from build123d import *

# Parameters (mm, degrees)
SKETCH_1_R      = 1.65
EXTRUDE_1_DEPTH = 1.6
EXTRUDE_2_DEPTH = 4.8
EXTRUDE_3_DEPTH = 0.01


with BuildPart() as part:
    # 草图1 → 凸台-拉伸1 (new body)
    with BuildSketch(Plane(origin=(0, 0, 0), x_dir=(1, 0, 0), z_dir=(0, 1, 0))):
        with BuildLine():
            Line((27.181335969, 0), (83.591335969, 0))
            Line((83.591335969, 0), (83.591335969, 96.2))
            Line((83.591335969, 96.2), (78.265479271, 96.2))
            ThreePointArc((78.265479271, 96.2), (76.9576214, 96.598857266), (76.026335969, 97.6))
            Line((76.026335969, 97.6), (55.386335969, 97.6))
            Line((55.386335969, 97.6), (34.746335969, 97.6))
            ThreePointArc((34.746335969, 97.6), (33.815050539, 96.598857266), (32.507192668, 96.2))
            Line((32.507192668, 96.2), (27.181335969, 96.2))
            Line((27.181335969, 96.2), (27.181335969, 0))
        make_face()
        with Locations(Location((31.021335969, 2.73, 0), (0, 0, 270))):
            Circle(SKETCH_1_R, mode=Mode.SUBTRACT)
        with Locations(Location((79.751335969, 2.73, 0), (0, 0, 90))):
            Circle(SKETCH_1_R, mode=Mode.SUBTRACT)
    extrude(amount=EXTRUDE_1_DEPTH)

    # 草图3 → 凸台-拉伸2 (add)
    with BuildSketch(Plane(origin=(0, 1.6, 0), x_dir=(1, 0, 0), z_dir=(0, 1, 0))):
        Polygon((55.386335969, 7), (27.886335969, 7), (27.886335969, 91.7), (82.886335969, 91.7), (82.886335969, 7), align=None)
    extrude(amount=EXTRUDE_2_DEPTH)

    # 草图4 → 凸台-拉伸3 (add)
    with BuildSketch(Plane(origin=(0, 6.4, 0), x_dir=(1, 0, 0), z_dir=(0, 1, 0))):
        Polygon((55.386335969, 88.95), (30.506335969, 88.95), (30.506335969, 14.51), (80.266335969, 14.51), (80.266335969, 88.95), align=None)
    extrude(amount=EXTRUDE_3_DEPTH)


solid = part.part
The listing builds one solid part. Answer for the finished solid, in the listing's coordinates (mm). A direction names the side the tool comes from. Coordinates: 2 decimals unless noted, no trailing zeros. Write each loop counter-clockwise with the first axis right and the second up, starting at its lowest first coordinate (ties: lowest second). Pieces come first, ordered by that corner, then holes. Notation, with made-up numbers: (56, 13.25) -> (65, 13.25) arc R30 cw to (65, 37.25) -> close; hole circle Ø3 at (-20, -26.75). An arc over 180 degrees is marked (long way). One line per question, with ' | ' between items.
1. Section D-D (y = 4.75) is taken. Determine the outline of the cut face in (x, z).
Verdict:
outline: (27.89, -91.7) -> (82.89, -91.7) -> (82.89, -7) -> (27.89, -7) -> close
2. Given pin 1 Ø1.4 at (y, z) = (4, -30.5) entering from +X; pin 2 Ø0.5 at (x, y) = (80.5, 1) entering from -Z; pin 3 Ø2.5 at (y, z) = (4.5, -51.5) entering from -X, each flat-ended and moving along its own axis, determine where each tip first touches the part or whether it passes through.
Verdict:
pin 1: stops at x = 82.89 | pin 2: stops at z = -96.2 | pin 3: stops at x = 27.89
3. Straight lines are drawn through the part: line 1 (X direction, y = 1.15, z = -2.73); line 2 (Z direction, x = 33.5, y = 2); line 3 (Y direction, x = 48, z = -10). For each, find the intervals that lie inside material, in ascending order.
Verdict:
line 1: x = 27.18 to 29.37, 32.67 to 78.1, 81.4 to 83.59 | line 2: z = -91.7 to -7 | line 3: y = 0 to 6.4
4. Which of the six approach directions +Z, -Z, +X, -X, +Y, -Y give full straight-line access (tool end or side, diameter ignored) to faces 1 (the flat face through (82.886, 4, -50)), 2 (the flat face through (55, 4, -91.7)), 3 (the flat face through (55, 4, -7))?
Verdict:
face 1: +Z, -Z, +X, +Y | face 2: -Z, +X, -X, +Y | face 3: +Z, +X, -X, +Y
5. Section A-A (z = -2.73) is taken. Determine the outline of the cut face in (x, y).
Verdict:
outline: (27.18, 0) -> (29.37, 0) -> (29.37, 1.6) -> (27.18, 1.6) -> close; (32.67, 0) -> (78.1, 0) -> (78.1, 1.6) -> (32.67, 1.6) -> close; (81.4, 0) -> (83.59, 0) -> (83.59, 1.6) -> (81.4, 1.6) -> close
